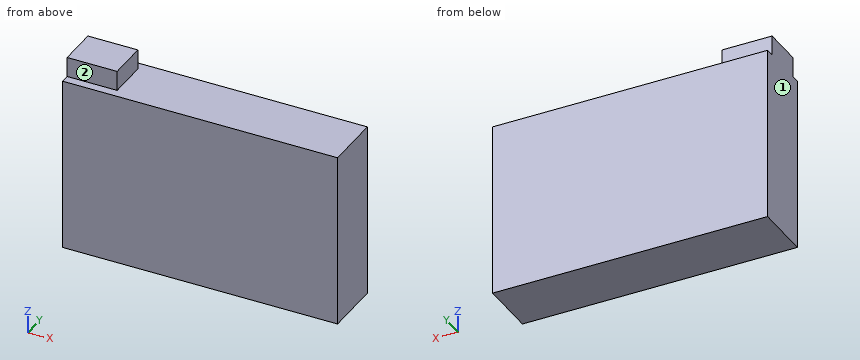
Autodesk Fusion 360 part; units mm, degrees
sketch "Sketch1" plane through (0, 0, 0) normal (0, 1, 0) x (1, 0, 0)
  line L0 (0, 0) -> (-55, 0)
  line L1 (-55, 0) -> (-55, -35)
  line L2 (-55, -35) -> (0, -35)
  line L3 (0, -35) -> (0, 0)
  dimension "d1" = 55
  dimension "d2" = 35
extrude "Extrude1" add sketch "Sketch1" along normal blind 11.5
sketch "Sketch2" plane through (0, 0, 35) normal (0, 0, 1) x (-1, 0, 0)
  line L0 (55, 0) -> (0, 0)
  line L1 (0, 0) -> (0, -11.5)
  line L2 (0, -11.5) -> (55, -11.5)
  line L3 (55, -11.5) -> (55, 0)
  line L4 (55, -9.75) -> (45, -9.75)
  line L5 (45, -9.75) -> (45, -1.75)
  line L6 (45, -1.75) -> (55, -1.75)
  line L7 (55, -1.75) -> (55, -9.75)
  line L8 (45, -5.75) -> (55, -5.75)
  dimension "d5" = 10
  dimension "d6" = 8
extrude "Extrude2" add sketch "Sketch2" along normal blind 4 contours L3 L5 L6 L7 L8 | L3 L4 L5 L7 L8
Model file for the job. Use its own axes, mm. Face numbers are marked on the shaded views. A direction names the side the tool comes from. Give positions to 0.01 mm unless a question says otherwise; leave off trailing zeros. Write each loop counter-clockwise with the first axis right and the second up, starting at its lowest first coordinate (ties: lowest second). Pieces come first, ordered by that corner, then holes. Notation, with made-up numbers: M 80.25,15 L 114.25,15 A6 cw 114.25,20 Z; hole C -21,0 d8. An arc over 180 degrees is marked long. Use a Markdown table: item, result.
1) Cut at A-A (x = -47.5). List the corners of the cut face in (y, z).
Responses:
| item | result |
|---|---|
| outline | M 0,0 L 11.5,0 L 11.5,35 L 9.75,35 L 9.75,39 L 1.75,39 L 1.75,35 L 0,35 Z |
2) Pin check, flat tips, straight feed: pin 1 (4.5 mm diameter, centred on y = 6.5, z = 37.5, fed in from +X); pin 2 (1 mm diameter, centred on x = -29.5, y = 2, fed in from +Z); pin 3 (1.2 mm diameter, centred on x = -48.5, z = 36.5, fed in from +Y). Stop position of each tip, or through.
Responses:
| item | result |
|---|---|
| pin 1 | stops at x = -45 |
| pin 2 | stops at z = 35 |
| pin 3 | stops at y = 9.75 |
3) Cut at B-B (y = 2.5). List the corners of the cut face in (x, z).
Responses:
| item | result |
|---|---|
| outline | M -55,0 L 0,0 L 0,35 L -45,35 L -45,39 L -55,39 Z |
4) Cut at C-C (x = -32). List the corners of the cut face in (y, z).
Responses:
| item | result |
|---|---|
| outline | M 0,0 L 11.5,0 L 11.5,35 L 0,35 Z |
5) Tool access for the marked faces 1 and 2: list every direction of +Z, -Z, +X, -X, +Y, -Y with a clear straight run to the whole face (end or side of a thin tool).
Responses:
| item | result |
|---|---|
| face 1 | +Z, -Z, -X, +Y, -Y |
| face 2 | +Z, +X, -X, -Y |
6) Drill centre lines: line 1 (Z direction, x = -29, y = 7.25); line 2 (X direction, y = 7.75, z = 35.5). Where is each one in solid material? Low to high. Write a range as from..to.
Responses:
| item | result |
|---|---|
| line 1 | z = 0..35 |
| line 2 | x = -55..-45 |
